Geometry: final body of the model. Coordinates: model frame, mm. Coordinates: 2 decimals unless noted, no trailing zeros. Loops run counter-clockwise (first coordinate to the right, second up) from the corner with the lowest first, then second, coordinate; pieces in that order, holes last. Notation, with made-up numbers: (-14.5, 11.5) - (23.5, 11.5) arc R35 cw to (23.5, 49.5) - close; hole circle Ø7 at (-9.5, 36.25). An arc over 180 degrees is marked (long way). Answer in a Markdown table with one row per item.
Autodesk Inventor part; units mm, degrees
ref_plane "YZ Plane" through (0, 0, 0) normal (1, 0, 0) x (0, 1, 0)
ref_plane "XZ Plane" through (0, 0, 0) normal (0, 1, 0) x (-1, 0, 0)
ref_plane "XY Plane" through (0, 0, 0) normal (0, 0, 1) x (1, 0, 0)
sketch "스케치1" plane through (0, 0, 0) normal (0, 1, 0) x (-1, 0, 0)
  line L0 (197, 1) -> (-93, 1)
  line L1 (-93, 1) -> (-93, 26)
  line L2 (-93, 26) -> (197, 26)
  line L3 (197, 26) -> (197, 1)
  point P0 (0, 0)
  dimension "d0" = 290
  dimension "d1" = 25
extrude "돌출1" add sketch "스케치1" along normal blind 2
sketch "스케치2" plane through (0, 0, 0) normal (0, -1, 0) x (1, 0, 0)
  line L0 (-197, 26) -> (93, 26)
  line L1 (93, 1) -> (-197, 1)
  line L2 (-154, 26) -> (-148.6, 26)
  line L3 (-148.6, 26) -> (-148.6, 1)
  line L4 (-148.6, 1) -> (-154, 1)
  line L5 (-154, 1) -> (-154, 26)
  line L6 (44.6, 26) -> (50, 26)
  line L7 (50, 26) -> (50, 1)
  line L8 (50, 1) -> (44.6, 1)
  line L9 (44.6, 1) -> (44.6, 26)
  line L10 (-197, 26) -> (-197, 1)
  line L11 (93, 1) -> (93, 26)
  point P0 (0, 0)
  dimension "d4" = 5.4
  dimension "d5" = 5.4
  dimension "d6" = 43
  dimension "d7" = 43
extrude "돌출2" cut sketch "스케치2" against normal blind 1 contours L0 L3 L1 L5 | L0 L7 L1 L9
sketch "스케치3" plane through (0, 0, 0) normal (0, -1, 0) x (1, 0, 0)
  line L0 (50, 26) -> (50, 1)
  line L1 (50, 1) -> (93, 1)
  line L2 (93, 1) -> (93, 26)
  line L3 (93, 26) -> (50, 26)
  line L4 (-154, 1) -> (-154, 26)
  line L5 (-154, 26) -> (-197, 26)
  line L6 (-197, 26) -> (-197, 1)
  line L7 (-197, 1) -> (-154, 1)
  line L8 (50, 1) -> (93, 1)
  line L9 (92, 1) -> (92, 26)
  line L10 (86.6, 1) -> (86.6, 26)
  line L11 (-196, 1) -> (-196, 26)
  line L12 (93, 1) -> (-197, 1)
  line L13 (-190.6, 1) -> (-190.6, 26)
  point P0 (0, 0)
  dimension "d10" = 1
  dimension "d11" = 5.4
  dimension "d12" = 1
  dimension "d13" = 5.4
extrude "돌출3" cut sketch "스케치3" against normal blind 1 contours L3 L9 L1 L10 | L7 L11 L5 L13
properties part number "앞판_중간" material "알루미늄 6061"
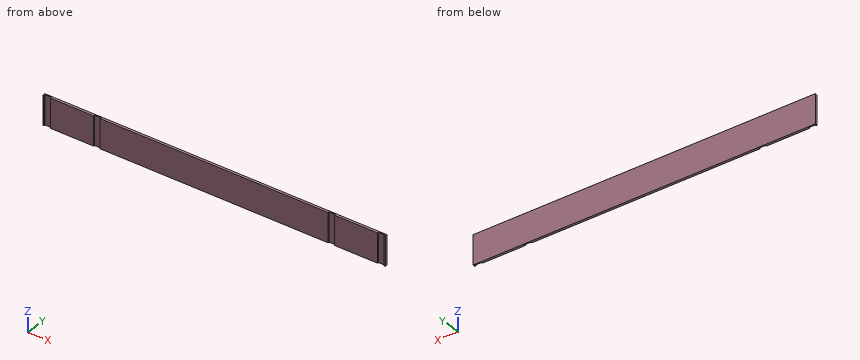
(1) First-contact query: pin 1 Ø4.5 at (x, z) = (47, 15.5) entering from -Y. Flat tip, straight axial feed; report the tip coordinate or a pass-through.
Verdict:
| item | result |
|---|---|
| pin 1 | stops at y = 1 |
(2) Ray query, probe 1 along X at (y, z) = (0.3, 2.5); probe 2 along Y at (x, z) = (45, 11). Return the intervals inside material, ascending.
Verdict:
| item | result |
|---|---|
| probe 1 | x = -197 to -196, -190.6 to -154, -148.6 to 44.6, 50 to 86.6, 92 to 93 |
| probe 2 | y = 1 to 2 |
(3) Cut plane B-B on z = 20. Output: boundary loops of the cut face in (x, y).
Verdict:
| item | result |
|---|---|
| outline | (-197, 0) - (-196, 0) - (-196, 1) - (-190.6, 1) - (-190.6, 0) - (-154, 0) - (-154, 1) - (-148.6, 1) - (-148.6, 0) - (44.6, 0) - (44.6, 1) - (50, 1) - (50, 0) - (86.6, 0) - (86.6, 1) - (92, 1) - (92, 0) - (93, 0) - (93, 2) - (-197, 2) - close |
(4) Cut plane A-A on y = 0.45. Output: boundary loops of the cut face in (x, z), then the cut area to 3 significant figures.
Verdict:
| item | result |
|---|---|
| outline | (-197, 1) - (-196, 1) - (-196, 26) - (-197, 26) - close; (-190.6, 1) - (-154, 1) - (-154, 26) - (-190.6, 26) - close; (-148.6, 1) - (44.6, 1) - (44.6, 26) - (-148.6, 26) - close; (50, 1) - (86.6, 1) - (86.6, 26) - (50, 26) - close; (92, 1) - (93, 1) - (93, 26) - (92, 26) - close |
| area | 6,710 mm² |
